Input: part model. Units: mm. Frame: model coordinates. A direction names the side the tool comes from. Round coordinates to 2 decimals unless told otherwise and drop trailing zeros. Loops run counter-clockwise (first coordinate to the right, second up) from the corner with the lowest first, then second, coordinate; pieces in that order, holes last. Notation, with made-up numbers: (-20, 89) -> (11, 89) arc R21 ccw to (11, 123) -> close; hole circle Ø3 at (-11.5, 16). An arc over 180 degrees is marked (long way). Answer as a JSON object with one key per item and string values.
```python
from build123d import *

# Parameters (mm, degrees)
BOSS_EXTRUDE1_DEPTH = 38.1
BOSS_EXTRUDE2_DEPTH = 19.05


with BuildPart() as part:
    # Sketch3 → Boss-Extrude1 (new body)
    with BuildSketch(Plane.XY):
        Polygon((0, 0), (0, 19.05), (-367.665, 19.05), (-374.65, 26.035), (-374.65, 41.275), (-381, 41.275), (-381, -22.225), (-374.65, -22.225), (-374.65, -6.985), (-367.665, 0), align=None)
    extrude(amount=BOSS_EXTRUDE1_DEPTH)

    # Sketch4 → Boss-Extrude2 (add)
    with BuildSketch(Plane(origin=(0, 19.05, 0), x_dir=(1, 0, 0), z_dir=(0, 1, 0))):
        Polygon((0, 0), (12.7, 12.7), (12.7, 31.75), (25.4, 31.75), (25.4, -69.85), (12.7, -69.85), (12.7, -50.8), (0, -38.1), align=None)
    extrude(amount=-BOSS_EXTRUDE2_DEPTH)


solid = part.part
```
1) Contact query for flat-ended pins moving along their axis: P1, Ø15, axis at y = 9.5, z = 60, coming from the -X side; P2, Ø10, axis at y = 22, z = -15.5, coming from the -X side; P3, Ø7.5, axis at y = 35, z = 21.5, coming from the +X side; P4, Ø1, axis at y = 21, z = 55, coming from the -X side. Output: stop coordinate, or through.
Output:
{"P1": "stops at x = 12.7", "P2": "stops at x = 11.46", "P3": "stops at x = -374.65", "P4": "passes through"}
2) Section A-A, the plane z = 23. Output: boundary loops of the cut face in (x, y) (3 decimals), plus the area to 3 significant figures.
Output:
{"outline": "(-381, -22.225) -> (-374.65, -22.225) -> (-374.65, -6.985) -> (-367.665, 0) -> (25.4, 0) -> (25.4, 19.05) -> (-367.665, 19.05) -> (-374.65, 26.035) -> (-374.65, 41.275) -> (-381, 41.275) -> close", "area": "8,070 mm^2"}
3) Ray query, probe 1 along Y at (x, z) = (-187, 21.5); probe 2 along X at (y, z) = (10, -18); probe 3 along Z at (x, y) = (-141.5, 1). Return the intervals inside material, ascending.
Output:
{"probe 1": "y = 0 to 19.05", "probe 2": "x = 12.7 to 25.4", "probe 3": "z = 0 to 38.1"}
4) Section C-C, the plane x = -41. Output: boundary loops of the cut face in (y, z), plus the area to 3 significant figures.
Output:
{"outline": "(0, 0) -> (19.05, 0) -> (19.05, 38.1) -> (0, 38.1) -> close", "area": "726 mm^2"}
5) Draft query along Y for faces 1 (the face through (-206, 7, 0)), 2 (the face through (-156, 0, 15)), 3 (the face through (-156, 19.05, 15)). Return one class per face: +Y half, -Y half, draft (parallel to the pull), parting line (faces both ways), or undercut.
Output:
{"face 1": "draft", "face 2": "-Y half", "face 3": "+Y half"}
6) Section D-D, the plane z = 47. Output: boundary loops of the cut face in (x, y).
Output:
{"outline": "(8.9, 0) -> (25.4, 0) -> (25.4, 19.05) -> (8.9, 19.05) -> close"}
7) Reachability of faces 4 (the face through (-374.65, 34, 19)), 5 (the face through (-374.65, -15, 19)), 6 (the face through (12.7, 10, -22)), 7 (the face through (12.7, 10, 60)) from +Z, -Z, +X, -X, +Y, -Y: full face, straight path, thin tool, end or side. Return the list, or none.
Output:
{"face 4": "+Z, -Z, +X, +Y", "face 5": "+Z, -Z, +X, -Y", "face 6": "-Z, -X, +Y, -Y", "face 7": "+Z, -X, +Y, -Y"}
8) Section B-B, the plane y = 15.5. Output: boundary loops of the cut face in (x, z), plus the area to 3 significant figures.
Output:
{"outline": "(-381, 0) -> (0, 0) -> (12.7, -12.7) -> (12.7, -31.75) -> (25.4, -31.75) -> (25.4, 69.85) -> (12.7, 69.85) -> (12.7, 50.8) -> (0, 38.1) -> (-381, 38.1) -> close", "area": "16,500 mm^2"}
